Design review of the part shown in the three views and the two pictorial views. Dimensions are in mm from the part's minimum x, y and z. Coordinates: 2 decimals unless noted, no trailing zeros. Write each loop counter-clockwise with the first axis right and the second up, starting at its lowest first coordinate (ties: lowest second). Pieces come first, ordered by that corner, then holes. Notation, with made-up numbers: (65, 46) - (108, 46) arc R23 ccw to (108, 80) - close; hole circle Ø6 at (77, -5). An arc over 180 degrees is marked (long way). Write each question's results on one line, items separated by ' | '.
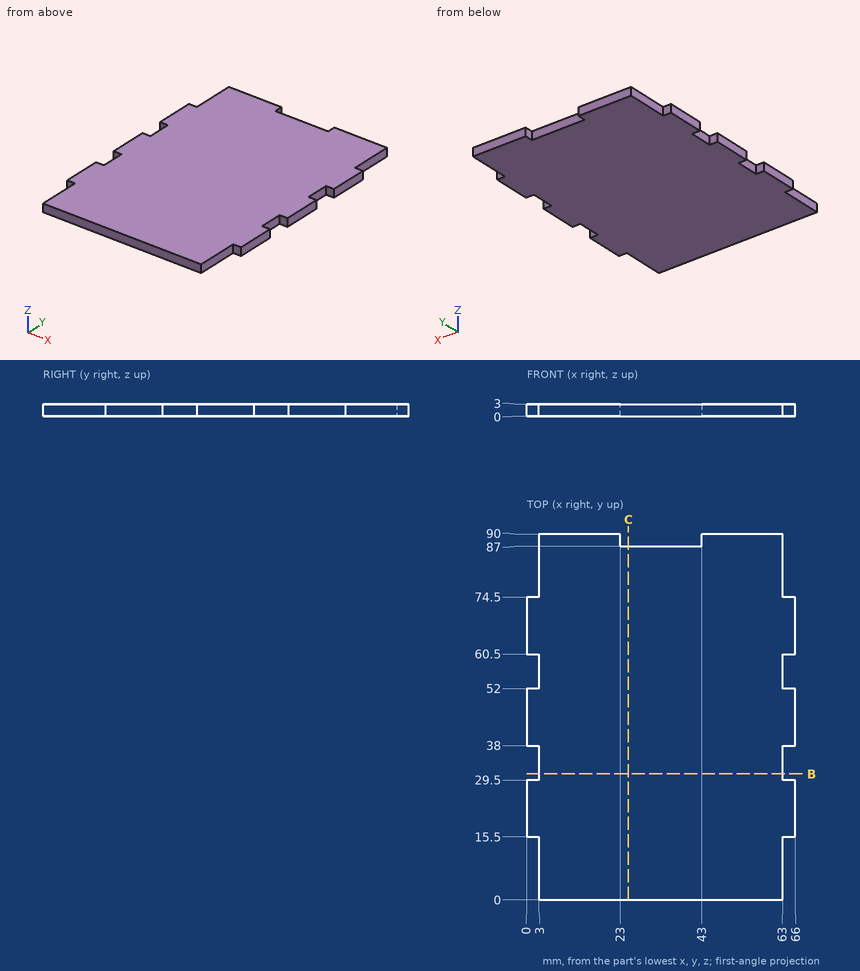
Q1. Wall thickness on line 1 along X through (y, z) = (4.5, 2.4); line 2 along Y through (x, z) = (39, 1.65): over which ranges is each line inside the solid? List them lowest first. Write a range as from..to.
Results found:
line 1: 3..63 | line 2: 0..87
Q2. For pin 1 (0.9 mm diameter, centred on y = 32, z = 2, fed in from -X); pin 2 (0.9 mm diameter, centred on x = 65, z = 2, fed in from +Y); pin 3 (1.5 mm diameter, centred on y = 7, z = 1, fed in from +X), all flat-tipped, find the tip position at first contact; note any pin that passes through.
Results found:
pin 1: x = 3 | pin 2: y = 74.5 | pin 3: x = 63
Q3. Take a section at B-B on y = 31. State the section outline as (x, z) points.
Results found:
outline: (3, 0) - (63, 0) - (63, 3) - (3, 3) - close
Q4. Take a section at C-C on x = 25. State the section outline as (y, z) points.
Results found:
outline: (0, 0) - (87, 0) - (87, 3) - (0, 3) - close
